Geometry: see drawing. Coordinates: mm, zero at the bounding-box minimum. A direction names the side the tool comes from. Coordinates: 2 decimals unless noted, no trailing zeros. Order: outer loops, then holes, each group sorted by start corner. A loop starts at its lowest first (then second) coordinate and runs counter-clockwise, first axis right, second up. Notation, with made-up numbers: (-6.75, 54) -> (48.25, 54) arc R26 ccw to (48.25, 92) -> close; hole circle Ø7 at (88, 34). An arc over 180 degrees is marked (long way). Write each question's results on one line, items separated by ' | '.
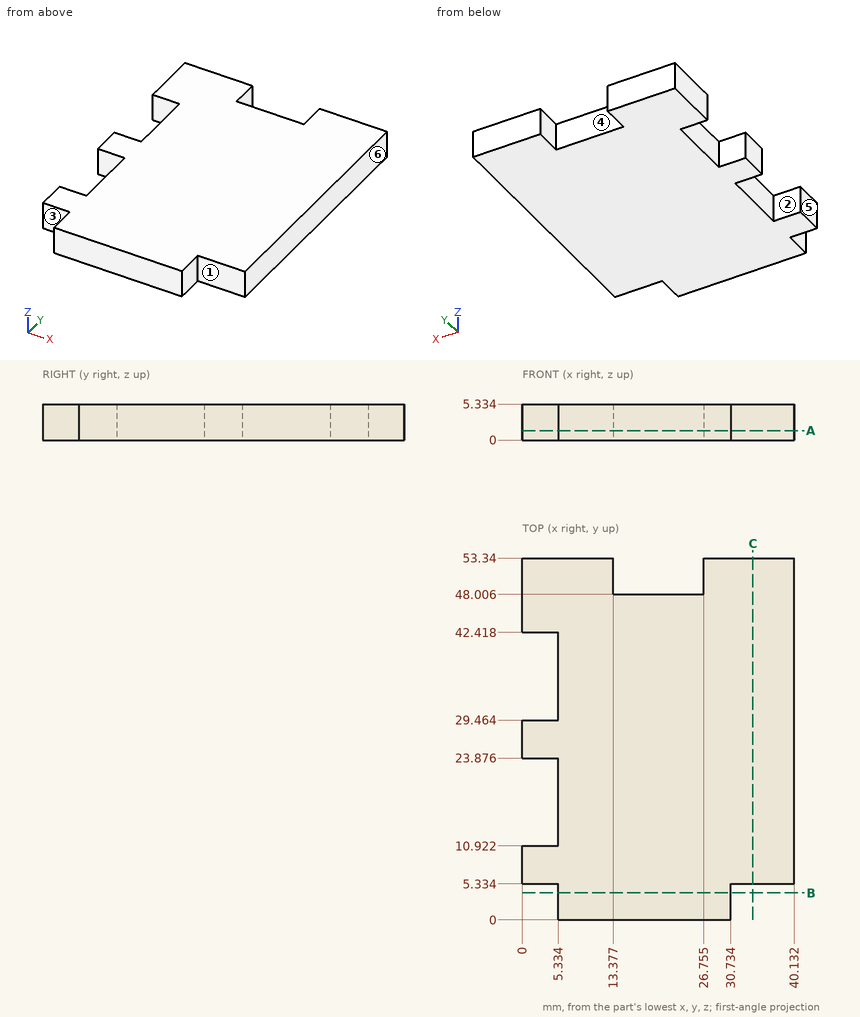
(1) Line query: line 1 along X through (y, z) = (50, 0.95) (1 decimal); line 2 along X through (y, z) = (32, 1.7); line 3 along Y through (x, z) = (20.5, 3.15). Output: solid intervals per line, ascending. Write a range as from..to.
Return value:
line 1: 0..13.4, 26.8..40.1 | line 2: 5.33..40.13 | line 3: 0..48.01
(2) Pin query (flat end, axial travel): P1, Ø2, axis at x = 4, y = 35, coming from the +Z side; P2, Ø3, axis at x = 23.5, y = 34, coming from the -Z side; P3, Ø2.5, axis at y = 20, z = 3, coming from the -X side; P4, Ø1.6, axis at x = 3.5, z = 2, coming from the -Y side. Return the tip coordinate at first contact, or that it passes through.
Return value:
P1: through | P2: z = 0 | P3: x = 5.33 | P4: y = 5.33
(3) Cut plane C-C, the plane x = 34. Return loops of the section in (y, z).
Return value:
outline: (5.33, 0) -> (53.34, 0) -> (53.34, 5.33) -> (5.33, 5.33) -> close
(4) Mould query, pull axis X, two halves, no side actions, for the marked faces 4, 5 and 6. Classes: +X half, -X half, draft (parallel to the pull), parting line (faces both ways), or undercut.
Return value:
face 4: undercut | face 5: -X half | face 6: +X half
(5) Reachability of the marked faces 1, 2 and 3 from +Z, -Z, +X, -X, +Y, -Y: full face, straight path, thin tool, end or side. Return the list, or none.
Return value:
face 1: +Z, -Z, +X, -Y | face 2: +Z, -Z, -X | face 3: +Z, -Z, -X, -Y
(6) Cut plane B-B, the plane y = 4. Return loops of the section in (x, z).
Return value:
outline: (5.33, 0) -> (30.73, 0) -> (30.73, 5.33) -> (5.33, 5.33) -> close
(7) Cut plane A-A, the plane z = 1.4. Return loops of the section in (x, y) (1 decimal).
Return value:
outline: (0, 5.3) -> (5.3, 5.3) -> (5.3, 0) -> (30.7, 0) -> (30.7, 5.3) -> (40.1, 5.3) -> (40.1, 53.3) -> (26.8, 53.3) -> (26.8, 48) -> (13.4, 48) -> (13.4, 53.3) -> (0, 53.3) -> (0, 42.4) -> (5.3, 42.4) -> (5.3, 29.5) -> (0, 29.5) -> (0, 23.9) -> (5.3, 23.9) -> (5.3, 10.9) -> (0, 10.9) -> close
